Work out the finished part from the listing and answer in its coordinate system (mm). A direction names the side the tool comes from. Give positions to 0.01 mm unless a question says otherwise; leave off trailing zeros. Answer in a Markdown table with one row per item. Add a question column.
Autodesk Inventor part; units mm, degrees
ref_plane "to_tube_XY" through (4.8006, 0, 0) normal (1, 0, 0) x (0, 0, -1)
ref_plane "to_tube_YZ" through (4.8006, 0, 0) normal (0, 0, -1) x (0, 1, 0)
ref_plane "to_tube_ZX" through (4.8006, 0, 0) normal (0, 1, 0) x (1, 0, 0)
sketch "Sketch_8" plane through (0, 0, 0) normal (0, 0, 1) x (1, 0, 0)
  line L0 (24.6126, 0) -> (0, 0)
  line L1 (0, 0) -> (0, 8.9091)
  line L2 (0, 8.9091) -> (0.762, 9.671)
  line L3 (0.762, 9.671) -> (4.0386, 9.671)
  line L4 (4.0386, 9.671) -> (4.8006, 8.9091)
  line L5 (4.8006, 8.9091) -> (5.5626, 8.9091)
  line L6 (5.5626, 8.9091) -> (5.5626, 10.3759)
  line L7 (5.5626, 10.3759) -> (8.7363, 10.3759)
  line L8 (8.7363, 10.3759) -> (9.3142, 10.9537)
  line L9 (9.3142, 10.9537) -> (23.8506, 10.9537)
  line L10 (23.8506, 10.9537) -> (24.6126, 10.1918)
  line L11 (24.6126, 10.1918) -> (24.6126, 0)
  line L12 (24.6126, 0) -> (0, 0)
revolve "Revolution1" add sketch "Sketch_8" angle 360 about axis through (24.6126, 0, 0) along (1, 0, 0)
sketch "Sketch_13" plane through (0, 0, 0) normal (0, 0, 1) x (1, 0, 0)
  line L0 (23.7253, 0) -> (0, 0)
  line L1 (0, 0) -> (0, 3.9624)
  line L2 (0, 3.9624) -> (21.4376, 3.9624)
  line L3 (21.4376, 3.9624) -> (23.7253, 0)
  line L4 (23.7253, 0) -> (0, 0)
revolve "Revolution2" cut sketch "Sketch_13" angle 360 about axis through (23.7253, 0, 0) along (1, 0, 0)
sketch "Sketch_19" plane through (0, 0, 0) normal (0, 1, 0) x (-1, 0, 0)
  line L0 (-17.4752, 10.9537) -> (-17.4752, 0)
  line L1 (-17.4752, 0) -> (-22.04, 0)
  line L2 (-22.04, 0) -> (-22.04, 2.1565)
  line L3 (-22.04, 2.1565) -> (-22.2949, 10.3187)
  line L4 (-22.2949, 10.3187) -> (-22.9299, 10.9537)
  line L5 (-22.9299, 10.9537) -> (-17.4752, 10.9537)
  line L6 (-17.4752, 10.9537) -> (-17.4752, 0)
revolve "Revolution3" cut sketch "Sketch_19" angle 360 about axis through (17.4752, 0, 10.9537) along (0, 0, 1)
sketch "Sketch_24" plane through (0, 0, 0) normal (0, 0, 1) x (1, 0, 0)
  line L0 (5.5626, 0) -> (4.8006, 0)
  line L1 (4.4955, 10.2917) -> (5.4401, 9.3472)
  arc A0 (5.4401, 9.1676) -> (5.4401, 9.3472) centre (5.3503, 9.2574) ccw
  line L2 (5.4401, 9.1676) -> (5.1816, 8.9091)
  line L3 (5.1816, 8.9091) -> (4.8006, 8.9091)
  line L4 (4.8006, 8.9091) -> (4.8006, 8.655)
  line L5 (4.8006, 8.655) -> (5.5626, 8.655)
  line L6 (5.5626, 8.655) -> (5.5626, 9.512)
  line L7 (5.5626, 9.512) -> (4.6987, 10.3759)
  line L8 (4.6987, 10.3759) -> (4.4955, 10.3759)
  line L9 (4.4955, 10.3759) -> (4.4955, 10.2917)
revolve "Revolution4" add sketch "Sketch_24" angle 360 about axis through (5.5626, 0, 0) along (1, 0, 0)
ref_plane "to_tube_XY" through (4.8006, 0, 0) normal (1, 0, 0) x (0, 0, -1)
ref_plane "to_tube_YZ" through (4.8006, 0, 0) normal (0, 0, -1) x (0, 1, 0)
ref_plane "to_tube_ZX" through (4.8006, 0, 0) normal (0, 1, 0) x (1, 0, 0)
ref_plane "to_nut_XY" through (27.0002, 0, 0) normal (1, 0, 0) x (0, 0, -1)
ref_plane "to_nut_YZ" through (27.0002, 0, 0) normal (0, 0, -1) x (0, 1, 0)
ref_plane "to_nut_ZX" through (27.0002, 0, 0) normal (0, 1, 0) x (1, 0, 0)
ref_plane "lovra1_XY" through (35.7124, 0, 0) normal (1, 0, 0) x (0, 0, -1)
ref_plane "lovra1_YZ" through (35.7124, 0, 0) normal (0, 0, -1) x (0, 1, 0)
ref_plane "lovra1_ZX" through (35.7124, 0, 0) normal (0, 1, 0) x (1, 0, 0)
ref_plane "lovra2_XY" through (35.7124, 7.874, 0) normal (1, 0, 0) x (0, 0, -1)
ref_plane "lovra2_YZ" through (35.7124, 7.874, 0) normal (0, 0, -1) x (0, 1, 0)
ref_plane "lovra2_ZX" through (35.7124, 7.874, 0) normal (0, 1, 0) x (1, 0, 0)
ref_plane "lovra3_XY" through (35.7124, -7.874, 0) normal (1, 0, 0) x (0, 0, -1)
ref_plane "lovra3_YZ" through (35.7124, -7.874, 0) normal (0, 0, -1) x (0, 1, 0)
ref_plane "lovra3_ZX" through (35.7124, -7.874, 0) normal (0, 1, 0) x (1, 0, 0)
ref_plane "olen_XY" through (24.6126, 0, 0) normal (1, 0, 0) x (0, 0, -1)
ref_plane "olen_YZ" through (24.6126, 0, 0) normal (0, 0, -1) x (0, 1, 0)
ref_plane "olen_ZX" through (24.6126, 0, 0) normal (0, 1, 0) x (1, 0, 0)
ref_plane "port2_XY" through (24.6126, 0, 0) normal (1, 0, 0) x (0, 0, -1)
ref_plane "port2_YZ" through (24.6126, 0, 0) normal (0, 0, -1) x (0, 1, 0)
ref_plane "port2_ZX" through (24.6126, 0, 0) normal (0, 1, 0) x (1, 0, 0)
ref_plane "port_XY" through (17.4752, 0, 0) normal (0, 0, 1) x (1, 0, 0)
ref_plane "port_YZ" through (17.4752, 0, 0) normal (1, 0, 0) x (0, 1, 0)
ref_plane "port_ZX" through (17.4752, 0, 0) normal (0, 1, 0) x (0, 0, 1)
ref_plane "lovra21_XY" through (0, 0, 5.2705) normal (1, 0, 0) x (0, 0, -1)
ref_plane "lovra21_YZ" through (0, 0, 5.2705) normal (0, 0, -1) x (0, 1, 0)
ref_plane "lovra21_ZX" through (0, 0, 5.2705) normal (0, 1, 0) x (1, 0, 0)
ref_plane "lovra22_XY" through (0, 0, -5.2705) normal (1, 0, 0) x (0, 0, -1)
ref_plane "lovra22_YZ" through (0, 0, -5.2705) normal (0, 0, -1) x (0, 1, 0)
ref_plane "lovra22_ZX" through (0, 0, -5.2705) normal (0, 1, 0) x (1, 0, 0)
ref_plane "to_screw_XY" through (17.4752, 2.032, -6.0452) normal (0, 1, 0) x (1, 0, 0)
ref_plane "to_screw_YZ" through (17.4752, 2.032, -6.0452) normal (1, 0, 0) x (0, 0, -1)
ref_plane "to_screw_ZX" through (17.4752, 2.032, -6.0452) normal (0, 0, -1) x (0, 1, 0)
ref_plane "to_mounting_bracket_XY" through (24.6126, 0, 0) normal (1, 0, 0) x (0, 0, -1)
ref_plane "to_mounting_bracket_YZ" through (24.6126, 0, 0) normal (0, 0, -1) x (0, 1, 0)
ref_plane "to_mounting_bracket_ZX" through (24.6126, 0, 0) normal (0, 1, 0) x (1, 0, 0)
properties part number "04PQ0000_rear_head"
(1) The mould has two halves that part along Y. Classify faces 4 (the face through (16.68, 5.05, -9.72)), 5 (the face through (0, 2, -4)), 6 (the face through (12.546, 0.06, 10.429)), 7 (the face through (22.405, -0.06, 10.429)): pulls with the +Y half, pulls with the -Y half, needs draft (parallel to the pull), parting line crosses it, or undercut.
(2) Which of the six approach directions +Z, -Z, +X, -X, +Y, -Y give full straight-line access (tool end or side, diameter ignored) to faces 1 (the face through (17.427, -4.565, 1.093)), 2 (the face through (4.994, -1.931, -8.697)), 3 (the face through (7.172, -10.366, 0.456))?
(3) Consider line 1 along Z through (x, y) = (11.25, 0); line 2 along Z through (x, y) = (6.5, 0); line 3 along Z through (x, y) = (15.25, 0). Determine where each line is inside the solid, lowest interval first. Write a range as from..to.
(4) Each of these flat-tipped pins is pushed along its axis until it touches: P1, Ø12, axis at x = 5, z = -4.5, coming from the +Y side; P2, Ø12, axis at x = 2.5, y = -4, coming from the -Z side; P3, Ø8, axis at x = 2.5, y = 1.5, coming from the +Z side. Where does it stop, or does it pass through?
Numbers:
| question | item | result |
|---|---|---|
| 1 | face 4 | parting line crosses it |
| 1 | face 5 | needs draft |
| 1 | face 6 | undercut |
| 1 | face 7 | undercut |
| 2 | face 1 | +Z |
| 2 | face 2 | none |
| 2 | face 3 | -X |
| 3 | line 1 | z = -10.95..-3.96, 3.96..10.95 |
| 3 | line 2 | z = -10.38..-3.96, 3.96..10.38 |
| 3 | line 3 | z = -10.95..-3.96 |
| 4 | P1 | stops at y = 10.95 |
| 4 | P2 | stops at z = -10.38 |
| 4 | P3 | stops at z = 10.38 |
